from build123d import *

# Parameters (mm, degrees)
SKETCH1_W           = 40
SKETCH1_H           = 20
BOSS_EXTRUDE1_DEPTH = 14
SKETCH2_W           = 54
SKETCH2_H           = 20
BOSS_EXTRUDE2_DEPTH = 1
SKETCH3_W           = 40
SKETCH3_H           = 20
BOSS_EXTRUDE3_DEPTH = 2.75
SKETCH4_R           = 3
BOSS_EXTRUDE4_DEPTH = 15.5
SKETCH5_R           = 1.673571511
SKETCH5_R_2         = 1.749374088
CUT_EXTRUDE3_DEPTH  = 9.5


with BuildPart() as part:
    # Sketch1 → Boss-Extrude1 (new, symmetric)
    with BuildSketch(Plane(origin=(0, 0, 0), x_dir=(1, 0, 0), z_dir=(0, 1, 0))):
        with Locations((2.196078431, 1.058823529)):
            Rectangle(SKETCH1_W, SKETCH1_H)
    extrude(amount=BOSS_EXTRUDE1_DEPTH, both=True)

    # Sketch2 → Boss-Extrude2 (add, symmetric)
    with BuildSketch(Plane.XZ.offset(14)):
        with Locations((2.196078431, -1.058823529)):
            Rectangle(SKETCH2_W, SKETCH2_H)
    extrude(amount=BOSS_EXTRUDE2_DEPTH, both=True)

    # Sketch3 → Boss-Extrude3 (add, symmetric)
    with BuildSketch(Plane.XZ.offset(15)):
        with Locations((2.196078431, -1.058823529)):
            Rectangle(SKETCH3_W, SKETCH3_H)
    extrude(amount=BOSS_EXTRUDE3_DEPTH, both=True)

    # Sketch4 → Boss-Extrude4 (add, symmetric)
    with BuildSketch(Plane.XZ.offset(17.75)):
        with Locations(Location((13.196078431, -1.058823529, 0), (0, 0, 270))):
            Circle(SKETCH4_R)
    extrude(amount=BOSS_EXTRUDE4_DEPTH, both=True)

    # Sketch5 → Cut-Extrude3 (cut)
    with BuildSketch(Plane.XZ.offset(15)):
        with Locations(Location((-22.803921569, 3.941176471, 0), (0, 0, 270))):
            Circle(SKETCH5_R)
        with Locations(Location((-22.803921569, -6.058823529, 0), (0, 0, 270))):
            Circle(SKETCH5_R_2)
    cut_extrude3 = extrude(amount=-CUT_EXTRUDE3_DEPTH, mode=Mode.SUBTRACT)

    # Mirror1: Cut-Extrude3 across plane
    add(cut_extrude3.mirror(Plane.ZY.offset(-2.196078431)), mode=Mode.SUBTRACT)


solid = part.part
Check sheet for the modelled part. Datum: model origin and axes. Units: mm. A direction names the side the tool comes from. Round coordinates to 2 decimals unless told otherwise and drop trailing zeros. Loops run counter-clockwise (first coordinate to the right, second up) from the corner with the lowest first, then second, coordinate; pieces in that order, holes last. Notation, with made-up numbers: M -16,-6.5 L 39,-6.5 A17 cw 39,-1.5 Z; hole C -10.5,72.25 d5. An arc over 180 degrees is marked long. One line per item, written item: value.
(1) Access from +Z, -Z, +X, -X, +Y, -Y to the whole of each face (thin tool, end or side, straight path). Record for faces 1 (the face through (-21, -15, -1)), 2 (the face through (26, -15, -1)), 3 (the face through (26, -13, -1)), 4 (the face through (-21, -13, -1)), 5 (the face through (16.17, -25.61, -0.67)).
Computed values:
face 1: +Z, -Z, -X, -Y
face 2: +Z, -Z, +X, -Y
face 3: +Z, -Z, +X, +Y
face 4: +Z, -Z, -X, +Y
face 5: -Y
(2) Sectioned sample at B-B, the plane x = 14. Record the cut outline in (y, z).
Computed values:
outline: M -33.25,-3.95 L -17.75,-3.95 L -17.75,-11.06 L 14,-11.06 L 14,8.94 L -17.75,8.94 L -17.75,1.83 L -33.25,1.83 Z
(3) Depth check by flat-ended pin: pin 1 Ø7.5 at (x, z) = (-22, -4.5) entering from +Y; pin 2 Ø12 at (y, z) = (3.5, 3) entering from -X; pin 3 Ø4 at (x, z) = (0, -7.5) entering from -Y; pin 4 Ø3 at (y, z) = (-16, 3.5) entering from +X. Enter the tip coordinate at first touch or a pass-through.
Computed values:
pin 1: stops at y = -13
pin 2: stops at x = -17.8
pin 3: stops at y = -17.75
pin 4: stops at x = 29.2
(4) Sectioned sample at A-A, the plane z = -8.75. Record the cut outline in (x, y).
Computed values:
outline: M -24.8,-15 L -17.8,-15 L -17.8,-17.75 L 22.2,-17.75 L 22.2,-15 L 29.2,-15 L 29.2,-13 L 22.2,-13 L 22.2,14 L -17.8,14 L -17.8,-13 L -24.8,-13 Z
(5) Sectioned sample at C-C, the plane z = 3.75. Record the cut outline in (x, y).
Computed values:
outline: M -24.8,-15 L -24.47,-15 L -24.47,-13 L -24.8,-13 Z; M -21.14,-15 L -17.8,-15 L -17.8,-17.75 L 22.2,-17.75 L 22.2,-15 L 25.53,-15 L 25.53,-13 L 22.2,-13 L 22.2,14 L -17.8,14 L -17.8,-13 L -21.14,-13 Z; M 28.86,-15 L 29.2,-15 L 29.2,-13 L 28.86,-13 Z
(6) Sectioned sample at D-D, the plane y = 3. Record the cut outline in (x, z).
Computed values:
outline: M -17.8,-11.06 L 22.2,-11.06 L 22.2,8.94 L -17.8,8.94 Z
(7) Release check for a two-part mould opening along X. For faces 6 (the face through (2, -17.75, -1)), 7 (the face through (25.537, -14.014, 4.159)), 8 (the face through (22.196, 1, -1)) record: +X half, -X half, draft (parallel to the pull), parting line (faces both ways), or undercut.
Computed values:
face 6: draft
face 7: undercut
face 8: +X half
(8) Thickness scan on line 1 (Z direction, x = 26.5, y = -13.5); line 2 (Y direction, x = -19, z = 6.5); line 3 (X direction, y = -9, z = 2). Record the ranges inside material, lowest first.
Computed values:
line 1: z = -11.06 to -7.66, -4.45 to 2.42, 5.46 to 8.94
line 2: y = -15 to -13
line 3: x = -17.8 to 22.2
